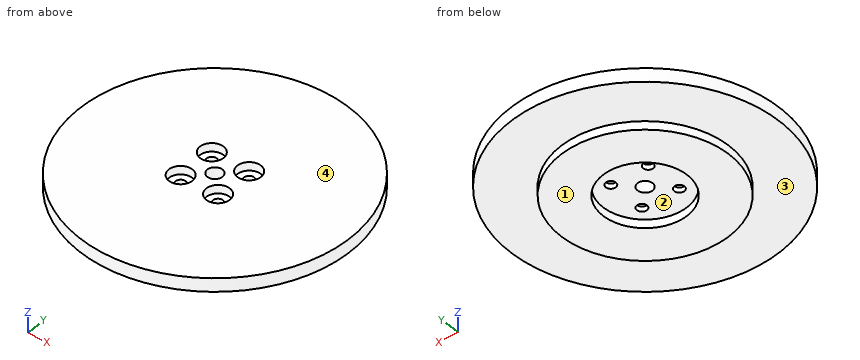
from build123d import *

# Parameters (mm, degrees)
SKETCH1_R           = 25
SKETCH1_R_2         = 12.5
BOSS_EXTRUDE1_DEPTH = 2.5
SKETCH2_R           = 40
SKETCH2_R_2         = 2.25
SKETCH2_R_3         = 1.5
BOSS_EXTRUDE2_DEPTH = 4
SKETCH3_R           = 3.5
CUT_EXTRUDE1_DEPTH  = 2.5


with BuildPart() as part:
    # Sketch1 → Boss-Extrude1 (new body)
    with BuildSketch(Plane.XY):
        Circle(SKETCH1_R)
        Circle(SKETCH1_R_2, mode=Mode.SUBTRACT)
    extrude(amount=BOSS_EXTRUDE1_DEPTH)

    # Sketch2 → Boss-Extrude2 (add)
    with BuildSketch(Plane.XY.offset(2.5)):
        Circle(SKETCH2_R)
        Circle(SKETCH2_R_2, mode=Mode.SUBTRACT)
        with Locations((-5.655999742, 5.657708628)):
            Circle(SKETCH2_R_3, mode=Mode.SUBTRACT)
        with Locations((-5.655999742, -5.657708628)):
            Circle(SKETCH2_R_3, mode=Mode.SUBTRACT)
        with Locations((5.655999742, -5.657708628)):
            Circle(SKETCH2_R_3, mode=Mode.SUBTRACT)
        with Locations((5.655999742, 5.657708628)):
            Circle(SKETCH2_R_3, mode=Mode.SUBTRACT)
    extrude(amount=BOSS_EXTRUDE2_DEPTH)

    # Sketch3 → Cut-Extrude1 (cut)
    with BuildSketch(Plane.XY.offset(6.5)):
        with Locations((-5.655999742, 5.657708628)):
            Circle(SKETCH3_R)
        with Locations((5.655999742, 5.657708628)):
            Circle(SKETCH3_R)
        with Locations((5.655999742, -5.657708628)):
            Circle(SKETCH3_R)
        with Locations((-5.655999742, -5.657708628)):
            Circle(SKETCH3_R)
    extrude(amount=-CUT_EXTRUDE1_DEPTH, mode=Mode.SUBTRACT)


solid = part.part
Design review of the part built by this model. Coordinates are the model's own, in mm. Face numbers are marked on the shaded views. A direction names the side the tool comes from. Round coordinates to 2 decimals unless told otherwise and drop trailing zeros. Write each loop counter-clockwise with the first axis right and the second up, starting at its lowest first coordinate (ties: lowest second). Pieces come first, ordered by that corner, then holes. Notation, with made-up numbers: (29, 68.25) -> (35, 68.25) arc R21 ccw to (35, 85.25) -> close; hole circle Ø3 at (59, 8). An arc over 180 degrees is marked (long way). One line per item, written item: value. Start each with the question number.
Q1. The part is to be moulded in two halves that separate along Y. For the marked faces 1 and 2, say which applies: pulls with the +Y half, pulls with the -Y half, needs draft (parallel to the pull), parting line crosses it, or undercut.
Q2. Add section D-D (x = 23). Give the boundary of the cut face in (y, z), then the cut area to 3 significant figures.
Q3. Tool access review of the marked faces 3 and 4: name each direction out of +Z, -Z, +X, -X, +Y, -Y from which nothing blocks a thin tool from reaching the whole face with its end or side.
Q4. Add section A-A (y = 0). Give the boundary of the cut face in (x, z), then the cut area to 4 significant figures.
Q5. Add section C-C (z = 1.5). Give the boundary of the cut face in (x, y), then the cut area to 3 significant figures.
Q6. To check wall thickness, follow probe 1 along Y at (x, z) = (0, 0.8); probe 2 along Z at (x, y) = (-20, -20); probe 3 along X at (y, z) = (-3.5, 0.5). State the ranges of each line that lie inside material, in increasing order.
Q7. Insertion check: P1, Ø2.5, axis at x = 0, y = 0, coming from the -Z side; P2, Ø5.5, axis at x = 5.66, y = 5.66, coming from the +Z side; P3, Ø1.5, axis at y = -11.5, z = 2.5, coming from the -X side; P4, Ø2, axis at x = -19, z = 1, coming from the +Y side. Each pin has a flat end and moves straight along its axis. Give the tip position at first contact, or say it passes through.
Q8. Add section B-B (x = 5.5). Give the boundary of the cut face in (y, z), then the cut area to 3 significant figures.
Response:
1. face 1: needs draft
1. face 2: undercut
2. outline: (-32.73, 2.5) -> (-9.8, 2.5) -> (-9.8, 0) -> (9.8, 0) -> (9.8, 2.5) -> (32.73, 2.5) -> (32.73, 6.5) -> (-32.73, 6.5) -> close
2. area: 311 mm^2
3. face 3: -Z
3. face 4: +Z, +X, -X, +Y, -Y
4. outline: (-40, 2.5) -> (-25, 2.5) -> (-25, 0) -> (-12.5, 0) -> (-12.5, 2.5) -> (-2.25, 2.5) -> (-2.25, 6.5) -> (-40, 6.5) -> close; (2.25, 2.5) -> (12.5, 2.5) -> (12.5, 0) -> (25, 0) -> (25, 2.5) -> (40, 2.5) -> (40, 6.5) -> (2.25, 6.5) -> close
4. area: 364.5 mm^2
5. outline: circle Ø50 at (0, 0); hole circle Ø25 at (0, 0)
5. area: 1,470 mm^2
6. probe 1: y = -25 to -12.5, 12.5 to 25
6. probe 2: z = 2.5 to 6.5
6. probe 3: x = -24.75 to -12, 12 to 24.75
7. P1: passes through
7. P2: stops at z = 4
7. P3: stops at x = -38.53
7. P4: stops at y = 17.35
8. outline: (-39.62, 2.5) -> (-24.39, 2.5) -> (-24.39, 0) -> (-11.22, 0) -> (-11.22, 2.5) -> (-7.15, 2.5) -> (-7.15, 4) -> (-9.15, 4) -> (-9.15, 6.5) -> (-39.62, 6.5) -> close; (-4.17, 2.5) -> (4.17, 2.5) -> (4.17, 4) -> (2.16, 4) -> (2.16, 6.5) -> (-2.16, 6.5) -> (-2.16, 4) -> (-4.17, 4) -> close; (7.15, 2.5) -> (11.22, 2.5) -> (11.22, 0) -> (24.39, 0) -> (24.39, 2.5) -> (39.62, 2.5) -> (39.62, 6.5) -> (9.15, 6.5) -> (9.15, 4) -> (7.15, 4) -> close
8. area: 339 mm^2
